Part model, mm, in its own coordinate system. Face numbers are marked on the shaded views. Give positions to 0.01 mm unless a question says otherwise; leave off trailing zeros. Write each loop counter-clockwise with the first axis right and the second up, starting at its lowest first coordinate (ties: lowest second). Pieces come first, ordered by that corner, then holes. Notation, with made-up numbers: M 11,61.5 L 57,61.5 A24 cw 57,96.5 Z; hole C 21.25,67 d5. An arc over 180 degrees is marked long. Use a Markdown table: item, result.
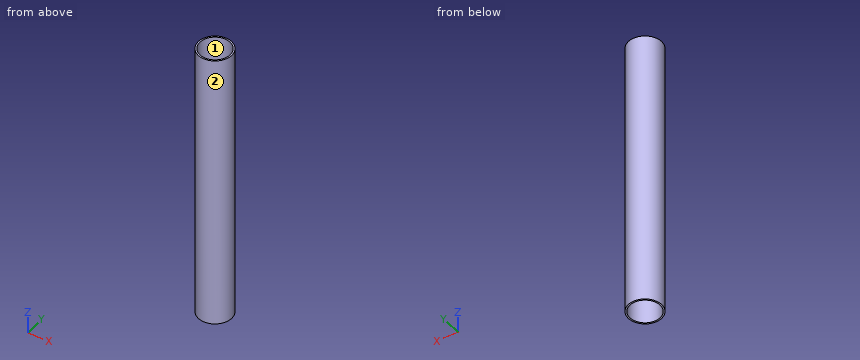
```python
from build123d import *

# Parameters (mm, degrees)
ESQUISSE1_R             = 19.2405
ESQUISSE1_R_2           = 17.4625
BOSS_EXTRU_1_DEPTH      = 914.4
ENL_V_START             = -63.5
ESQUISSE3_R             = 19.2405
ENL_V_MAT_EXTRU_1_DEPTH = 63.5
ENL_V_START_2           = -527.05
ESQUISSE4_R             = 19.2405
ENL_V_MAT_EXTRU_2_DEPTH = 527.05


with BuildPart() as part:
    # Esquisse1 → Boss.-Extru.1 (new body)
    with BuildSketch(Plane.XY):
        Circle(ESQUISSE1_R)
        Circle(ESQUISSE1_R_2, mode=Mode.SUBTRACT)
    extrude(amount=BOSS_EXTRU_1_DEPTH)

    # Esquisse3 → Enlèv. mat.-Extru.1 (cut)
    with BuildSketch(Plane.XY.offset(914.4).offset(ENL_V_START)):
        Circle(ESQUISSE3_R)
    extrude(amount=ENL_V_MAT_EXTRU_1_DEPTH, mode=Mode.SUBTRACT)

    # Esquisse4 → Enlèv. mat.-Extru.2 (cut)
    with BuildSketch(Plane.XY.offset(850.9).offset(ENL_V_START_2)):
        Circle(ESQUISSE4_R)
    extrude(amount=ENL_V_MAT_EXTRU_2_DEPTH, mode=Mode.SUBTRACT)


solid = part.part
```
1. Cut at C-C, the plane z = 186. Give the cut face in (x, y) (1 decimal).
Findings below:
| item | result |
|---|---|
| outline | C 0,0 d38.5; hole C 0,0 d34.9 |
2. Drop flat-ended pins along their axis: P1, Ø6, axis at y = -14.5, z = 107.5, coming from the +X side; P2, Ø3, axis at x = 2, z = 176.5, coming from the +Y side; P3, Ø6, axis at y = -13, z = 213.5, coming from the +X side. Give the stop position or say it passes through.
Findings below:
| item | result |
|---|---|
| P1 | x = 15.43 |
| P2 | y = 19.23 |
| P3 | x = 16.44 |
3. Two-plate mould, pull along X, no slides. Class the marked faces 1 and 2: released by +X, released by -X, zero draft, split by the parting line, or undercut.
Findings below:
| item | result |
|---|---|
| face 1 | undercut |
| face 2 | split by the parting line |
4. Cut at A-A, the plane x = 0. Give the cut face in (y, z), then the cut area to 3 significant figures.
Findings below:
| item | result |
|---|---|
| outline | M -19.24,0 L -17.46,0 L -17.46,323.85 L -19.24,323.85 Z; M 17.46,0 L 19.24,0 L 19.24,323.85 L 17.46,323.85 Z |
| area | 1,150 mm2 |
5. Drill centre lines: L1, parallel to Y at x = 0, z = 72.5; L2, parallel to Y at x = -1.5, z = 276.5; L3, parallel to X at y = -0.5, z = 110. Where is each one in solid material? Low to high.
Findings below:
| item | result |
|---|---|
| L1 | -19.24 to -17.46, 17.46 to 19.24 |
| L2 | -19.18 to -17.4, 17.4 to 19.18 |
| L3 | -19.23 to -17.46, 17.46 to 19.23 |
